Read the model definition and answer for the solid it produces. Units are mm, in the model's axes. A direction names the side the tool comes from. Coordinates: 2 decimals unless noted, no trailing zeros. Order: outer loops, then holes, each group sorted by start corner. A loop starts at its lowest first (then second) coordinate and runs counter-clockwise, first axis right, second up. Notation, with made-up numbers: M 79,16.5 L 122,16.5 A15 ccw 122,21.5 Z; hole C -2.75,7.25 d1. An arc over 180 degrees is marked long. Write each question's results on one line, items separated by ' | '.
```python
from build123d import *

# Parameters (mm, degrees)
F0_W     = 62.928204
F0_H     = 22
F1_DEPTH = 4
F2_DEPTH = 2
F3_R     = 1.5
F4_DEPTH = 2


with BuildPart() as f1:
    # F0 (on Top) → F1 (new body)
    with BuildSketch(Plane.XY):
        Rectangle(F0_W, F0_H)
        Polygon((-26.732051, -2), (26.732051, -2), (28.464102, -5), (26.732051, -8), (-26.732051, -8), (-28.464102, -5), align=None, mode=Mode.SUBTRACT)
        Polygon((-26.732051, 2), (-28.464102, 5), (-26.732051, 8), (26.732051, 8), (28.464102, 5), (26.732051, 2), align=None, mode=Mode.SUBTRACT)
    extrude(amount=-F1_DEPTH)

    # F0 (on Top) → F2 (join)
    with BuildSketch(Plane.XY):
        Polygon((28.464102, -5), (26.732051, -2), (-26.732051, -2), (-28.464102, -5), (-26.732051, -8), (26.732051, -8), align=None)
        with BuildLine():
            ThreePointArc((-25, -6.75), (-26.75, -5), (-25, -3.25))
            Line((-25, -3.25), (25, -3.25))
            ThreePointArc((25, -3.25), (26.75, -5), (25, -6.75))
            Line((25, -6.75), (-25, -6.75))
        make_face(mode=Mode.SUBTRACT)
        Polygon((-26.732051, 8), (-28.464102, 5), (-26.732051, 2), (26.732051, 2), (28.464102, 5), (26.732051, 8), align=None)
        with BuildLine():
            ThreePointArc((-25, 3.25), (-26.75, 5), (-25, 6.75))
            Line((-25, 6.75), (25, 6.75))
            ThreePointArc((25, 6.75), (26.75, 5), (25, 3.25))
            Line((25, 3.25), (-25, 3.25))
        make_face(mode=Mode.SUBTRACT)
    extrude(amount=-F2_DEPTH)

    # F3 (on Front) → F4 (join, symmetric)
    with BuildSketch(Plane.XZ):
        with BuildLine():
            Line((-5.5, -50.5), (-5.5, -25.5))
            ThreePointArc((-5.5, -25.5), (0, -20), (5.5, -25.5))
            Line((5.5, -25.5), (5.5, -50.5))
            Line((5.5, -50.5), (31.464102, -4))
            Line((31.464102, -4), (-31.464102, -4))
            Line((-31.464102, -4), (-5.5, -50.5))
        make_face()
        with Locations((-10.944086, -31)):
            Circle(F3_R, mode=Mode.SUBTRACT)
        with Locations((10.944086, -31)):
            Circle(F3_R, mode=Mode.SUBTRACT)
    extrude(amount=F4_DEPTH, both=True)


solid = f1.part
```
(1) For faces 4 (the cylindrical face through (26.75, 5.04, -0.99)), 5 (the flat face through (5.5, 0, -38)), 6 (the flat face through (0, 9, -4)), determine the directions among +Z, -Z, +X, -X, +Y, -Y from which every point of the face is accessible in a straight line to the end or side of a thin tool.
Conclusion:
face 4: +Z, -Z | face 5: -Z, +Y, -Y | face 6: -Z, +X, -X, +Y
(2) The part is cut by section B-B, the plane y = 0.5. Write down the section's boundary in (x, z), then the cut area to 3 significant figures.
Conclusion:
outline: M -31.46,-4 L -5.5,-50.5 L -5.5,-25.5 A5.5 cw 5.5,-25.5 L 5.5,-50.5 L 31.46,-4 L 31.46,0 L -31.46,0 Z; hole C -10.94,-31 d3; hole C 10.94,-31 d3 | area: 1,630 mm²
(3) The part is cut by section C-C, the plane z = -35.5. Write down the section's boundary in (x, y).
Conclusion:
outline: M -13.88,-2 L -5.5,-2 L -5.5,2 L -13.88,2 Z; M 5.5,-2 L 13.88,-2 L 13.88,2 L 5.5,2 Z
(4) The part is cut by section D-D, the plane y = 4.25. Write down the section's boundary in (x, z), then the cut area to 3 significant figures.
Conclusion:
outline: M -31.46,-4 L -28.03,-4 L -28.03,-2 L -26.58,-2 L -26.58,0 L -31.46,0 Z; M 26.58,-2 L 28.03,-2 L 28.03,-4 L 31.46,-4 L 31.46,0 L 26.58,0 Z | area: 33.3 mm²
(5) Straight lines are drawn through the part: line 1 (Y direction, x = 1, z = -4.5); line 2 (Z direction, x = 15, y = 7.75); line 3 (X direction, y = 3, z = -3). For each, find the intervals that lie inside material, in ascending order.
Conclusion:
line 1: -2 to 2 | line 2: -2 to 0 | line 3: -31.46 to -27.31, 27.31 to 31.46
(6) The mould has two halves that part along Y. Classify faces 1 (the flat face through (0, 0, 0)), 2 (the flat face through (27.6, -6.5, -3)), 3 (the flat face through (0, -11, -2)): pulls with the +Y half, pulls with the -Y half, needs draft (parallel to the pull), parting line crosses it, or undercut.
Conclusion:
face 1: needs draft | face 2: undercut | face 3: pulls with the -Y half
(7) The part is cut by section A-A, the plane x = 0. Write down the section's boundary in (y, z), then the cut area to 3 significant figures.
Conclusion:
outline: M -11,-4 L -8,-4 L -8,-2 L -6.75,-2 L -6.75,0 L -11,0 Z; M -3.25,-2 L -2,-2 L -2,-20 L 2,-20 L 2,-2 L 3.25,-2 L 3.25,0 L -3.25,0 Z; M 6.75,-2 L 8,-2 L 8,-4 L 11,-4 L 11,0 L 6.75,0 Z | area: 114 mm²
(8) Given pin 1 (10 mm diameter, centred on x = 11.5, y = -4.5, fed in from +Z); pin 2 (4 mm diameter, centred on x = 10.94, z = -31, fed in from -Y); pin 3 (4.5 mm diameter, centred on y = 0, z = -36.5, fed in from +X); pin 4 (12 mm diameter, centred on y = 1.5, z = -44, fed in from +X), each flat-ended and moving along its own axis, determine where each tip first touches the part or whether it passes through.
Conclusion:
pin 1: z = 0 | pin 2: y = -2 | pin 3: x = 14.57 | pin 4: x = 12.48
